Geometry check sheet. Reference: the model listing, model coordinates, mm. Give positions to 0.01 mm unless a question says otherwise; leave off trailing zeros. Loops run counter-clockwise (first coordinate to the right, second up) from the corner with the lowest first, then second, coordinate; pieces in that order, holes last. Notation, with made-up numbers: (15, -8) -> (25, -8) arc R16 ccw to (25, 2) -> close; hole circle Ø3 at (62, 18.5). An arc over 180 degrees is marked (long way). Write each question's results on one line, items separated by ' | '. Start each with the question number.
1) Scan lines: line 1 (X direction, y = -2, z = 61); line 2 (Y direction, x = -2.25, z = 49); line 3 (X direction, y = -34.05, z = 165.1). Record each from-to range of solid material in increasing order. Write a range as from..to.
2) Sectioned sample at B-B on z = 312. Record the cut outline in (x, y).
3) Sectioned sample at A-A on y = -23. Record the cut outline in (x, z).
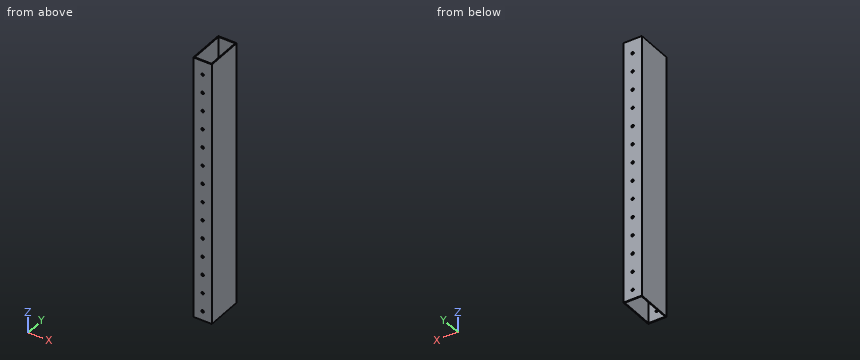
Autodesk Inventor part; units mm, degrees
ref_plane "YZ Plane" through (0, 0, 0) normal (1, 0, 0) x (0, 1, 0)
ref_plane "XZ Plane" through (0, 0, 0) normal (0, 1, 0) x (-1, 0, 0)
ref_plane "XY Plane" through (0, 0, 0) normal (0, 0, 1) x (1, 0, 0)
sketch "Sketch1" plane through (0, 0, 0) normal (0, 0, 1) x (1, 0, 0)
  line L0 (-12.1708, 16.0073) -> (13.2292, 16.0073)
  line L1 (13.2292, 16.0073) -> (13.2292, -34.7927)
  line L2 (13.2292, -34.7927) -> (-12.1708, -34.7927)
  line L3 (-12.1708, -34.7927) -> (-12.1708, 16.0073)
  line L4 (11.9592, 14.7373) -> (-10.9008, 14.7373)
  line L5 (-10.9008, 14.7373) -> (-10.9008, -33.5227)
  line L6 (-10.9008, -33.5227) -> (11.9592, -33.5227)
  line L7 (11.9592, -33.5227) -> (11.9592, 14.7373)
  point P0 (0, 0)
  dimension "d0" = 25.4
  dimension "d1" = 50.8
  dimension "d2" = 1.27
extrude "Extrusion1" add sketch "Sketch1" along normal blind 361.95
sketch "Sketch2" plane through (-12.1708, 16.0073, 0) normal (0, 1, 0) x (1, 0, 0)
  circle A0 centre (12.7, -12.7) radius 1.7272
  line L0 (25.4, 0) -> (0, 0)
  line L1 (0, 0) -> (0, -361.95)
  point P0 (12.1708, 0)
  dimension "d5" = 3.4544
  dimension "d6" = 12.7
  dimension "d7" = 12.7
extrude "Extrusion2" cut sketch "Sketch2" against normal through all
pattern_linear "Rectangular Pattern1" count 36 spacing 25.4 along (0, 0, 1) of "Extrusion2"
equation "\"d3\" = d13"
equation "\"d10\" = d14"
equation "\"d13\" = 361.95"
equation "\"d14\" = d13"
properties part number "TurretSupp"
Result:
1) line 1: -12.17..-10.9, 11.96..13.23 | line 2: -34.79..-33.52, 14.74..16.01 | line 3: -12.17..-1.2, 2.26..13.23
2) outline: (-12.17, -34.79) -> (13.23, -34.79) -> (13.23, 16.01) -> (-12.17, 16.01) -> close; hole (-10.9, -33.52) -> (11.96, -33.52) -> (11.96, 14.74) -> (-10.9, 14.74) -> close
3) outline: (-12.17, 0) -> (-10.9, 0) -> (-10.9, 361.95) -> (-12.17, 361.95) -> close; (11.96, 0) -> (13.23, 0) -> (13.23, 361.95) -> (11.96, 361.95) -> close
